from build123d import *

# Parameters (mm, degrees)
F0_R            = 104.775
F0_R_2          = 101.6
F1_DEPTH        = 101.6
F2_R            = 142.875
F2_R_2          = 101.6
F3_DEPTH        = 3.175
F5_D            = 9.921875
F5_COPIES_COUNT = 8


# Not quite as in the source:
# - a length typed as a fraction of an inch, garbled in the dataset ("3 / 203.2 mm" for 3/8 in), is restored
# - a pattern or mirror of a feature is missing from the dataset's text; its kind, count and spacing are read off the source's solid


with BuildPart() as f1:
    # F0 (on Top) → F1 (new body)
    with BuildSketch(Plane.XY):
        Circle(F0_R)
        Circle(F0_R_2, mode=Mode.SUBTRACT)
    extrude(amount=F1_DEPTH)

    # F2 (on face) → F3 (join)
    with BuildSketch(Plane(origin=(0, 0, 0), x_dir=(1, 0, 0), z_dir=(0, 0, -1))):
        Circle(F2_R)
        Circle(F2_R_2, mode=Mode.SUBTRACT)
    extrude(amount=F3_DEPTH)

    # F5 (through all)
    with Locations(Plane.XY):
        with Locations((117.3327006289, -48.6007959104)):
            f5 = Hole(F5_D / 2)

    # F5_copies: F5 ×8 about axis
    f5_copies_axis = Axis((0, 0, 0), (0, 0, 1))
    for i in range(1, F5_COPIES_COUNT):
        add(f5.rotate(f5_copies_axis, i * 360 / F5_COPIES_COUNT), mode=Mode.SUBTRACT)


solid = f1.part
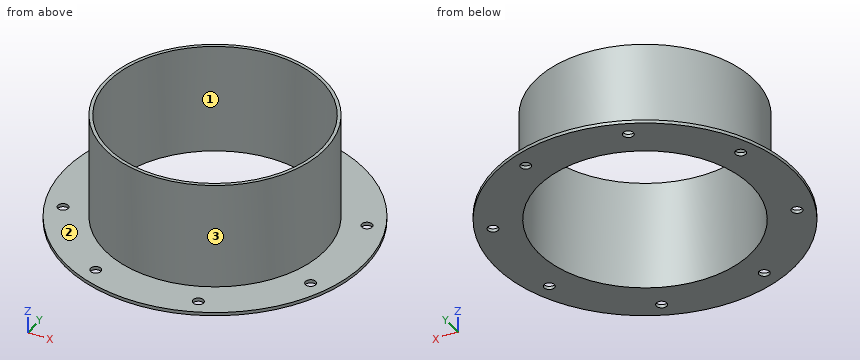
The listing builds one solid part. Answer for the finished solid, in the listing's coordinates (mm). Face numbers are marked on the shaded views. Round coordinates to 2 decimals unless told otherwise and drop trailing zeros. Order: outer loops, then holes, each group sorted by start corner. A loop starts at its lowest first (then second) coordinate and runs counter-clockwise, first axis right, second up. Notation, with made-up numbers: (1.25, -23.5) -> (20.25, -23.5) arc R30 ccw to (20.25, 15.5) -> close; hole circle Ø9 at (-10, -8.75). An arc over 180 degrees is marked (long way). Write each question's results on one line, items separated by ' | '. Start each with the question number.
Q1. Find section A-A (y = 0). Determine the outline of the cut face in (x, z) (3 decimals), then the cut area to 3 significant figures.
Q2. Find section C-C (z = 75.5). Determine the outline of the cut face in (x, y) (3 decimals).
Q3. Straight lines are drawn through the part: probe 1 along Z at (x, y) = (84.5, -107) (3 decimals); probe 2 along X at (y, z) = (78, 60); probe 3 along X at (y, z) = (-91, 84.5). For each, find the intervals that lie inside material, in ascending order. Write a range as from..to.
Q4. Find section B-B (x = 97.5). Determine the outline of the cut face in (y, z) (3 decimals).
Q5. The mould has two halves that part along Y. Classify the marked faces 1, 2 and 3: pulls with the +Y half, pulls with the -Y half, needs draft (parallel to the pull), parting line crosses it, or undercut.
Q6. Each of these flat-tipped pins is pushed along its axis until it touches: pin 1 (4 mm diameter, centred on x = -71, z = 31, fed in from -Y); pin 2 (1.5 mm diameter, centred on x = -97.5, y = -96.5, fed in from +Z); pin 3 (1.5 mm diameter, centred on x = 40.5, z = 39, fed in from +Y). Where does it stop, or does it pass through?
Worked answers:
1) outline: (-142.875, -3.175) -> (-101.6, -3.175) -> (-101.6, 101.6) -> (-104.775, 101.6) -> (-104.775, 0) -> (-142.875, 0) -> close; (101.6, -3.175) -> (142.875, -3.175) -> (142.875, 0) -> (104.775, 0) -> (104.775, 101.6) -> (101.6, 101.6) -> close | area: 907 mm2
2) outline: circle Ø209.55 at (0, 0); hole circle Ø203.2 at (0, 0)
3) probe 1: z = -3.175..0 | probe 2: x = -69.96..-65.1, 65.1..69.96 | probe 3: x = -51.93..-45.18, 45.18..51.93
4) outline: (-104.437, -3.175) -> (-28.571, -3.175) -> (-28.571, 101.6) -> (-38.361, 101.6) -> (-38.361, 0) -> (-104.437, 0) -> close; (28.571, -3.175) -> (104.437, -3.175) -> (104.437, 0) -> (38.361, 0) -> (38.361, 101.6) -> (28.571, 101.6) -> close
5) face 1: undercut | face 2: needs draft | face 3: parting line crosses it
6) pin 1: stops at y = -78.85 | pin 2: stops at z = 0 | pin 3: stops at y = 96.94
